Autodesk Inventor part; units mm, degrees
ref_plane "YZ Plane" through (0, 0, 0) normal (1, 0, 0) x (0, 1, 0)
ref_plane "XZ Plane" through (0, 0, 0) normal (0, 1, 0) x (-1, 0, 0)
ref_plane "XY Plane" through (0, 0, 0) normal (0, 0, 1) x (1, 0, 0)
sketch "Szkic1" plane through (0, 0, 0) normal (0, 1, 0) x (-1, 0, 0)
  line L0 (12.7, -3.666174) -> (12.7, -16)
  line L1 (0, -16) -> (0, 0)
  arc A0 (0, -16) -> (12.7, -16) centre (6.35, -16) ccw
  line L2 (0, 3.666174) -> (22.51666, 16.666174)
  line L3 (0, 0) -> (0, 3.666174)
  line L4 (22.51666, 16.666174) -> (55.316329, 63.508956)
  line L5 (65.71956, 56.224535) -> (31.304974, 7.075413)
  circle A1 centre (6.35, -16) radius 2.5
  circle A2 centre (6.35, 0) radius 2.5
  line L6 (65.71956, 56.224535) -> (55.316329, 63.508956)
  line L7 (22.51666, 16.666174) -> (28.86666, 5.667652)
  line L8 (31.304974, 7.075413) -> (12.7, -3.666174)
  line L9 (19.05, 0) -> (12.7, 10.998523)
  dimension "d5" = 155
  dimension "d7" = 5
  dimension "d9" = 26
  dimension "d11" = 12.7
  dimension "d13" = 60
extrude "Wyciągnięcie proste1" add sketch "Szkic1" against normal blind 3 contours L7 L4 L6 L5 L8
ref_plane "Płaszczyzna konstrukcyjna1" through (-15.875, -6.175, -1.833087) normal (-0.5, 0, -0.8660254) x (-0.8660254, 0, 0.5)
sketch "Szkic2" plane through (-15.875, -6.175, -1.833087) normal (-0.5, 0, -0.8660254) x (-0.8660254, 0, 0.5)
  line L0 (15.001477, 3.175) -> (11.826477, 0)
  line L1 (11.799797, -0.02668) -> (15.001477, 3.175)
  line L2 (12.880157, 5.29632) -> (10.583837, 3)
  line L3 (15.001477, 3.175) -> (15.001477, 6.175)
  line L4 (0, 6.175) -> (16.409238, 6.175)
  line L5 (12.880157, 5.29632) -> (13.758837, 6.175)
  line L6 (15.001477, 3.175) -> (11.826477, 0)
  line L7 (13.758837, 6.175) -> (15.001477, 6.175)
  line L8 (15.001477, 6.175) -> (15.001477, 3.175)
  line L9 (10.583837, 3) -> (0, 3)
  line L10 (10.583837, 3) -> (10.583837, 3)
  line L11 (0, 3) -> (0, 0)
  line L12 (0, 0) -> (11.826477, 0)
  line L13 (11.826477, 0) -> (11.826477, 0)
  point P0 (-12.83161, 6.175)
  dimension "d27" = 3
  dimension "d34" = 3.175
extrude "Wyciągnięcie proste3" add sketch "Szkic2" against normal blind 12.7
extrude "Wyciągnięcie proste4" add sketch "Szkic1" against normal blind 6.175 contours L0 A0 L1 L3 L2 L9 L8
extrude "Wyciągnięcie proste5" cut sketch "Szkic1" against normal blind 3.175 contours L0 A0 L1 L3 L2 L9 L8
fillet "Zaokrąglenie2" radius 1.5 4 edges at (-24.6155, 0, 10.5456) (-21.8659, -3.175, 8.9581) (-22.942, -6.175, 9.5794) (-25.6917, -3, 11.1669)
fillet "Zaokrąglenie3" radius 6.35 6 edges at (-12.7, -4.675, -3.6662) (-31.305, -1.5, 7.0754) (-65.7196, -1.5, 56.2245) (-22.5167, -1.5674, 16.6662) (0, -4.675, 3.6662) (-55.3163, -1.5, 63.509)
mirror "Odbij1" about plane through (-44.11811, 0, 34.588304) normal (0, 1, 0)
properties material "Stal nierdzewna"
Work out the finished part from the listing and answer in its coordinate system (mm). A direction names the side the tool comes from. Round coordinates to 2 decimals unless told otherwise and drop trailing zeros. Order: outer loops, then holes, each group sorted by start corner. A loop starts at its lowest first (then second) coordinate and runs counter-clockwise, first axis right, second up.
Q1. Find the intervals of material crossed by line 1 along Y through (x, z) = (-2.5, -1) (3 decimals); line 2 along Z through (x, y) = (-6.35, -5.5); line 3 along Z through (x, y) = (-5.5, 4.5), in increasing order.
Solution:
line 1: y = -6.175 to -3.175, 3.175 to 6.175
line 2: z = -22.35 to -18.5, -13.5 to -2.5, 2.5 to 7.33
line 3: z = -22.29 to -18.35, -13.65 to -2.35, 2.35 to 6.84
Q2. A tool of negligible diameter and unlimited length cuts with its end or side. For faces 1 (the flat face through (-12.7, -5, -12)), 2 (the cylindrical face through (-0.874, -4.654, 3.215)), 3 (the flat face through (-23.3, -1.57, 9.68)), from which of +Z, -Z, +X, -X, +Y, -Y can it reach the whole face along a straight path? Write none if from no direction.
Solution:
face 1: -Z, -X, +Y, -Y
face 2: +Z, +X, +Y, -Y
face 3: -Z, +X
Q3. The mould has two halves that part along Y. Classify faces 4 (the flat face through (-24.357, -4.571, 10.336)), 5 (the cylindrical face through (-25.688, 3.117, 11.252)), 6 (the flat face through (-47.305, 0.042, 29.925)), 7 (the cylindrical face through (-21.774, 3.064, 9.008)): pulls with the +Y half, pulls with the -Y half, needs draft (parallel to the pull), parting line crosses it, or undercut.
Solution:
face 4: pulls with the -Y half
face 5: pulls with the +Y half
face 6: needs draft
face 7: undercut
Q4. Given pin 1 Ø5 at (x, y) = (-18.5, -3) entering from -Z; pin 2 Ø4 at (y, z) = (0.5, 18.5) entering from +X; pin 3 Ø20 at (x, z) = (-45.5, 32) entering from -Y, each flat-ended and moving along its own axis, determine where each tip first touches the part or whether it passes through.
Solution:
pin 1: stops at z = -1.76
pin 2: stops at x = -22.09
pin 3: stops at y = -3
Q5. A cutting plane is placed at C-C, the plane z = 48. Determine the outline of the cut face in (x, y).
Solution:
outline: (-59.96, -3) - (-44.46, -3) - (-44.46, 3) - (-59.96, 3) - close
Q6. A cutting plane is placed at A-A, the plane x = -6.35. Determine the outline of the cut face in (y, z) (3 decimals), then the cut area to 3 significant figures.
Solution:
outline: (-6.175, -22.35) - (-3.175, -22.35) - (-3.175, -18.5) - (-6.175, -18.5) - close; (-6.175, -13.5) - (-3.175, -13.5) - (-3.175, -2.5) - (-6.175, -2.5) - close; (-6.175, 2.5) - (-3.175, 2.5) - (-3.175, 7.332) - (-6.175, 7.332) - close; (3.175, -22.35) - (6.175, -22.35) - (6.175, -18.5) - (3.175, -18.5) - close; (3.175, -13.5) - (6.175, -13.5) - (6.175, -2.5) - (3.175, -2.5) - close; (3.175, 2.5) - (6.175, 2.5) - (6.175, 7.332) - (3.175, 7.332) - close
area: 118 mm2
Q7. A cutting plane is placed at D-D, the plane x = -44. Determine the outline of the cut face in (y, z), then the cut area to 3 significant figures.
Solution:
outline: (-3, 25.21) - (3, 25.21) - (3, 47.35) - (-3, 47.35) - close
area: 133 mm2
Q8. A cutting plane is placed at B-B, the plane y = 1.75. Determine the outline of the cut face in (x, z).
Solution:
outline: (-62.08, 51.02) - (-32.11, 8.23) arc R6.35 ccw to (-30.09, 6.37) - (-26.27, 4.17) - (-19.92, 15.17) - (-21.3, 15.96) arc R6.35 cw to (-23.32, 17.82) - (-51.67, 58.31) arc R6.35 ccw to start
